from build123d import *

# Parameters (mm, degrees)
SKETCH_1_R      = 4
SKETCH_1_R_2    = 5.1
SKETCH_1_R_3    = 1.5
EXTRUDE_1_DEPTH = 5


with BuildPart() as part:
    # 草图1 → 凸台-拉伸1 (new body)
    with BuildSketch(Plane(origin=(0, 0, 0), x_dir=(0, 0, -1), z_dir=(1, 0, 0))):
        Polygon((-37.5, 105), (-55, 105), (-55, 75), (-50, 75), (-50, 35), (-55, 35), (-55, 0), (-37.5, 0), (-37.5, 5), (-17.5, 5), (-17.5, 0), (0, 0), (0, 35), (-5, 35), (-5, 75), (0, 75), (0, 105), (-17.5, 105), (-17.5, 100), (-37.5, 100), align=None)
        with Locations((-27.5, 16)):
            Circle(SKETCH_1_R, mode=Mode.SUBTRACT)
        with Locations((-27.5, 80)):
            Circle(SKETCH_1_R_2, mode=Mode.SUBTRACT)
        with Locations((-2.5, 90)):
            Circle(SKETCH_1_R_3, mode=Mode.SUBTRACT)
        with Locations((-52.5, 90)):
            Circle(SKETCH_1_R_3, mode=Mode.SUBTRACT)
        with Locations((-52.5, 17.5)):
            Circle(SKETCH_1_R_3, mode=Mode.SUBTRACT)
        with Locations((-2.5, 17.5)):
            Circle(SKETCH_1_R_3, mode=Mode.SUBTRACT)
        with BuildLine():
            ThreePointArc((-31.944781032, 88.677927263), (-34.397440233, 86.891140561), (-36.181985067, 84.436849703))
            ThreePointArc((-36.181985067, 84.436849703), (-35.420037694, 82.082187052), (-33.065375043, 82.844134425))
            ThreePointArc((-33.065375043, 82.844134425), (-31.921436047, 84.417397795), (-30.34921861, 85.562773886))
            ThreePointArc((-30.34921861, 85.562773886), (-29.589423133, 87.918131785), (-31.944781032, 88.677927263))
        make_face(mode=Mode.SUBTRACT)
        with BuildLine():
            ThreePointArc((-18.822072737, 84.444781032), (-20.608859439, 86.897440233), (-23.063150297, 88.681985067))
            ThreePointArc((-23.063150297, 88.681985067), (-25.417812948, 87.920037694), (-24.655865575, 85.565375043))
            ThreePointArc((-24.655865575, 85.565375043), (-23.082602205, 84.421436047), (-21.937226114, 82.84921861))
            ThreePointArc((-21.937226114, 82.84921861), (-19.581868215, 82.089423133), (-18.822072737, 84.444781032))
        make_face(mode=Mode.SUBTRACT)
        with BuildLine():
            ThreePointArc((-23.055218968, 71.322072737), (-20.602559767, 73.108859439), (-18.818014933, 75.563150297))
            ThreePointArc((-18.818014933, 75.563150297), (-19.579962306, 77.917812948), (-21.934624957, 77.155865575))
            ThreePointArc((-21.934624957, 77.155865575), (-23.078563953, 75.582602205), (-24.65078139, 74.437226114))
            ThreePointArc((-24.65078139, 74.437226114), (-25.410576867, 72.081868215), (-23.055218968, 71.322072737))
        make_face(mode=Mode.SUBTRACT)
        with BuildLine():
            ThreePointArc((-36.177927263, 75.555218968), (-34.391140561, 73.102559767), (-31.936849703, 71.318014933))
            ThreePointArc((-31.936849703, 71.318014933), (-29.582187052, 72.079962306), (-30.344134425, 74.434624957))
            ThreePointArc((-30.344134425, 74.434624957), (-31.917397795, 75.578563953), (-33.062773886, 77.15078139))
            ThreePointArc((-33.062773886, 77.15078139), (-35.418131785, 77.910576867), (-36.177927263, 75.555218968))
        make_face(mode=Mode.SUBTRACT)
    extrude(amount=EXTRUDE_1_DEPTH)


solid = part.part
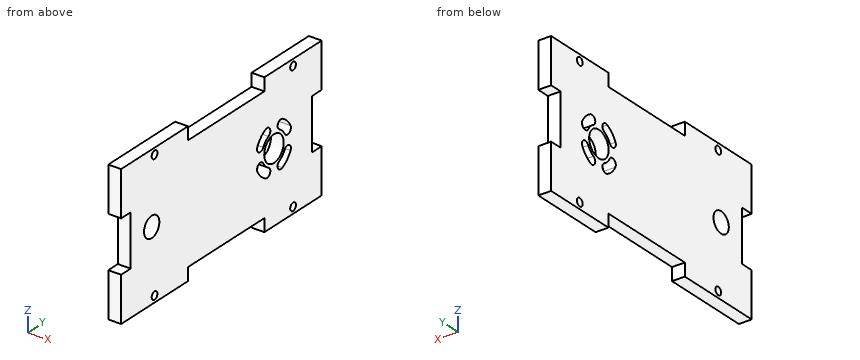
Verification items for the finished model (mm, model axes). Give positions to 0.01 mm unless a question says otherwise; leave off trailing zeros. Write each loop counter-clockwise with the first axis right and the second up, starting at its lowest first coordinate (ties: lowest second). Pieces come first, ordered by that corner, then holes. Notation, with made-up numbers: (29, 1.25) - (77, 1.25) arc R22 ccw to (77, 31.25) - close; hole circle Ø3 at (-32, -5). An arc over 180 degrees is marked (long way). Answer as CSV lines item,"result". Start each with the question number.
1. Sectioned sample at A-A (y = 80). Record the boundary of the cut face in (x, z), then the cut area to 3 significant figures.
2. Thickness scan on line 1 (Z direction, x = 1.95, y = 90); line 2 (Y direction, x = 2.15, z = 52.5); line 3 (Y direction, x = 3.2, z = 27.5). Record the ranges inside material, lowest first.
3. Depth check by flat-ended pin: pin 1 (2.5 mm diameter, centred on y = 90, z = 52.5, fed in from -X). Enter the tip coordinate at first touch or a pass-through.
4. Sectioned sample at C-C (x = 1.8). Count the separate pieces of the cut face and the enclosed holes in it, then the cut area to 3 significant figures.
5. Sectioned sample at D-D (y = 17.5). Record the boundary of the cut face in (x, z).
6. Sectioned sample at B-B (z = 2.5). Record the boundary of the cut face in (x, y).
Derived:
1,outline,"(0, 0) - (5, 0) - (5, 22.4) - (0, 22.4) - close; (0, 32.6) - (5, 32.6) - (5, 55) - (0, 55) - close"
1,area,"224 mm²"
2,line 1,"0 to 1, 4 to 51, 54 to 55"
2,line 2,"0 to 16, 19 to 35, 75 to 88.5, 91.5 to 105"
2,line 3,"5 to 12, 20 to 74.9, 85.1 to 100"
3,pin 1,"through"
4,separate pieces,"1"
4,enclosed holes,"10"
4,area,"4,910 mm²"
5,outline,"(0, 0) - (5, 0) - (5, 1) - (0, 1) - close; (0, 4) - (5, 4) - (5, 23.79) - (0, 23.79) - close; (0, 31.21) - (5, 31.21) - (5, 51) - (0, 51) - close; (0, 54) - (5, 54) - (5, 55) - (0, 55) - close"
6,outline,"(0, 0) - (5, 0) - (5, 16) - (0, 16) - close; (0, 19) - (5, 19) - (5, 35) - (0, 35) - close; (0, 75) - (5, 75) - (5, 88.5) - (0, 88.5) - close; (0, 91.5) - (5, 91.5) - (5, 105) - (0, 105) - close"
